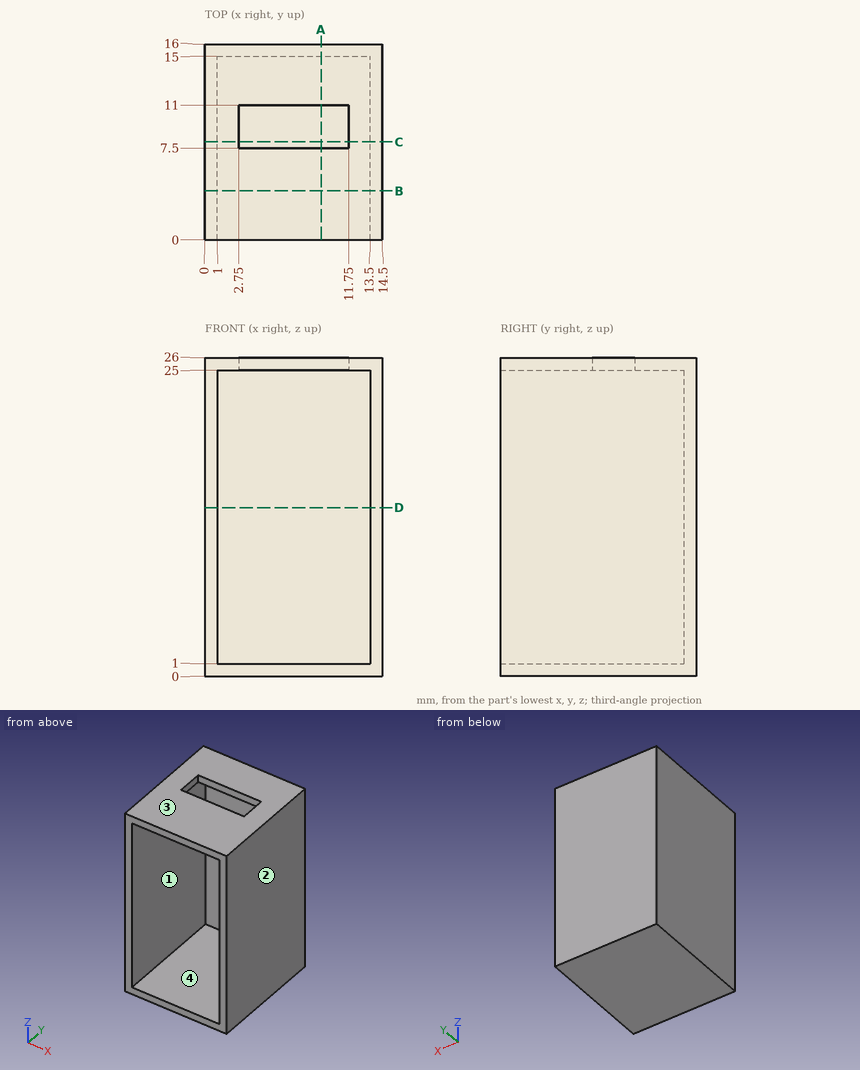
Geometry: see drawing. Coordinates: mm, zero at the bounding-box minimum. Give positions to 0.01 mm unless a question says otherwise; leave off trailing zeros. Order: outer loops, then holes, each group sorted by start corner. A loop starts at its lowest first (then second) coordinate and runs counter-clockwise, first axis right, second up.
Q1. Ray query, probe 1 along X at (y, z) = (4, 1.75); probe 2 along Z at (x, y) = (10, 2.5); probe 3 along Y at (x, z) = (12.25, 3.5). Return the intervals inside material, ascending.
Checked values:
probe 1: x = 0 to 1, 13.5 to 14.5
probe 2: z = 0 to 1, 25 to 26
probe 3: y = 15 to 16
Q2. Section A-A on x = 9.5. Output: boundary loops of the cut face in (y, z).
Checked values:
outline: (0, 0) - (16, 0) - (16, 26) - (11, 26) - (11, 25) - (15, 25) - (15, 1) - (0, 1) - close; (0, 25) - (7.5, 25) - (7.5, 26) - (0, 26) - close
Q3. Section C-C on y = 8. Output: boundary loops of the cut face in (x, z).
Checked values:
outline: (0, 0) - (14.5, 0) - (14.5, 26) - (11.75, 26) - (11.75, 25) - (13.5, 25) - (13.5, 1) - (1, 1) - (1, 25) - (2.75, 25) - (2.75, 26) - (0, 26) - close
Q4. Section D-D on z = 13.75. Output: boundary loops of the cut face in (x, y), and give its area (3 significant figures).
Checked values:
outline: (0, 0) - (1, 0) - (1, 15) - (13.5, 15) - (13.5, 0) - (14.5, 0) - (14.5, 16) - (0, 16) - close
area: 44.5 mm2
Q5. Section B-B on y = 4. Output: boundary loops of the cut face in (x, z).
Checked values:
outline: (0, 0) - (14.5, 0) - (14.5, 26) - (0, 26) - close; hole (1, 1) - (13.5, 1) - (13.5, 25) - (1, 25) - close
Q6. Contact query for flat-ended pins moving along their axis: pin 1 Ø1 at (x, y) = (8.5, 13.5) entering from -Z; pin 2 Ø6 at (x, z) = (6, 12.5) entering from -Y. Output: stop coordinate, or through.
Checked values:
pin 1: stops at z = 0
pin 2: stops at y = 15
Q7. Draft query along Z for the marked faces 1, 2, 3 and 4. Return one class per face: +Z half, -Z half, draft (parallel to the pull), parting line (faces both ways), or undercut.
Checked values:
face 1: undercut
face 2: draft
face 3: +Z half
face 4: undercut
